The listing builds one solid part. Answer for the finished solid, in the listing's coordinates (mm). Round coordinates to 2 decimals unless told otherwise and drop trailing zeros. One line per item, written item: value. Start each with the question number.
1. Straight lines are drawn through the part: line 1 (Z direction, x = 196, y = -171); line 2 (Y direction, x = -143, z = 23); line 3 (Y direction, x = 56, z = 24). For each, find the intervals that lie inside material, in ascending order.
2. A flat-ended cylindrical pin translates along its axis: P1, Ø6, axis at x = 44.5, y = -13, coming from the +Z side. Find the tip coordinate at first contact, or state that the pin passes through.
3. For a pull along X with two mould halves and no side action, classify faces 1 (the flat face through (-3, 250, 12)), 2 (the flat face through (-3, 3, 20)), 3 (the flat face through (-250, -3, 12)) as released by +X, released by -X, zero draft, split by the parting line, or undercut.
from build123d import *

# Parameters (mm, degrees)
F0_W     = 500
F0_H     = 500
F1_DEPTH = 25
F2_W     = 490.0000095367
F2_H     = 490.0000095367
F3_DEPTH = 5
F4_SIZE  = 4.99999


# Not quite as in the source:
# - a fillet or chamfer is up to 0.001 mm smaller than in the source, because OpenCascade refuses the exact size


with BuildPart() as f1:
    # F0 (on Top) → F1 (new body)
    with BuildSketch(Plane.XY):
        Rectangle(F0_W, F0_H)
    extrude(amount=F1_DEPTH)

    # F2 (on face) → F3 (cut)
    with BuildSketch(Plane.XY.offset(25)):
        Rectangle(F2_W, F2_H)
    extrude(amount=-F3_DEPTH, mode=Mode.SUBTRACT)

    # F4 (size 5 in the source; OpenCascade refuses exactly that, so slightly less here)
    f4_edges = [f1.edges().sort_by_distance(p)[0] for p in [
        (0, -245.000005, 20),
        (245.000005, 0, 20),
        (0, 245.000005, 20),
        (-245.000005, 0, 20),
    ]]
    chamfer(f4_edges, length=F4_SIZE)


solid = f1.part
Answer list:
1. line 1: z = 0 to 20
1. line 2: y = -250 to -243, 243 to 250
1. line 3: y = -250 to -244, 244 to 250
2. P1: stops at z = 20
3. face 1: zero draft
3. face 2: undercut
3. face 3: released by -X
